Here's the drawing with two shaded views (mm, measured from the low corner). I have some questions. A direction names the side the tool comes from. Give positions to 0.01 mm unless a question says otherwise; leave off trailing zeros. Loops run counter-clockwise (first coordinate to the right, second up) from the corner with the lowest first, then second, coordinate; pieces in that order, holes last. Notation, with made-up numbers: (48, 26.25) - (64, 26.25) arc R14 cw to (64, 40.25) - close; hole circle Ø11 at (-28.75, 46). An arc over 180 degrees is marked (long way). Answer as a JSON object with one key per item and string values. Group by question number.
Item 1: Suppose I cut it at B-B on z = 21. Write out the boundary of the cut face in (x, y), and give its area (3 significant figures).
Item 2: Which directions (+Z, -Z, +X, -X, +Y, -Y) give clear straight access to the entire face, cutting with the end or side of a thin tool? Please do the marked faces 1, 2, 3, 4 and 5.
Item 3: Suppose I cut it at A-A on z = 7.5. Write out the boundary of the cut face in (x, y), and give its area (3 significant figures).
Item 4: Please list where these lines run through material, in increasing order: L1, parallel to Z at x = 22.5, y = 25; L2, parallel to X at y = 5, z = 81; L3, parallel to X at y = 10, z = 60.5.
Item 5: Will these pins go through, and if not, where does the flat tip stop? pin 1 (1 mm diameter, centred on x = 29.5, z = 21.5, fed in from +Y); pin 2 (10 mm diameter, centred on x = 19, z = 55.5, fed in from +Y); pin 3 (1 mm diameter, centred on x = 31, y = 37.5, fed in from -Z).
Item 6: Suppose I cut it at C-C on z = 68. Write out the boundary of the cut face in (x, y), and give its area (3 significant figures).
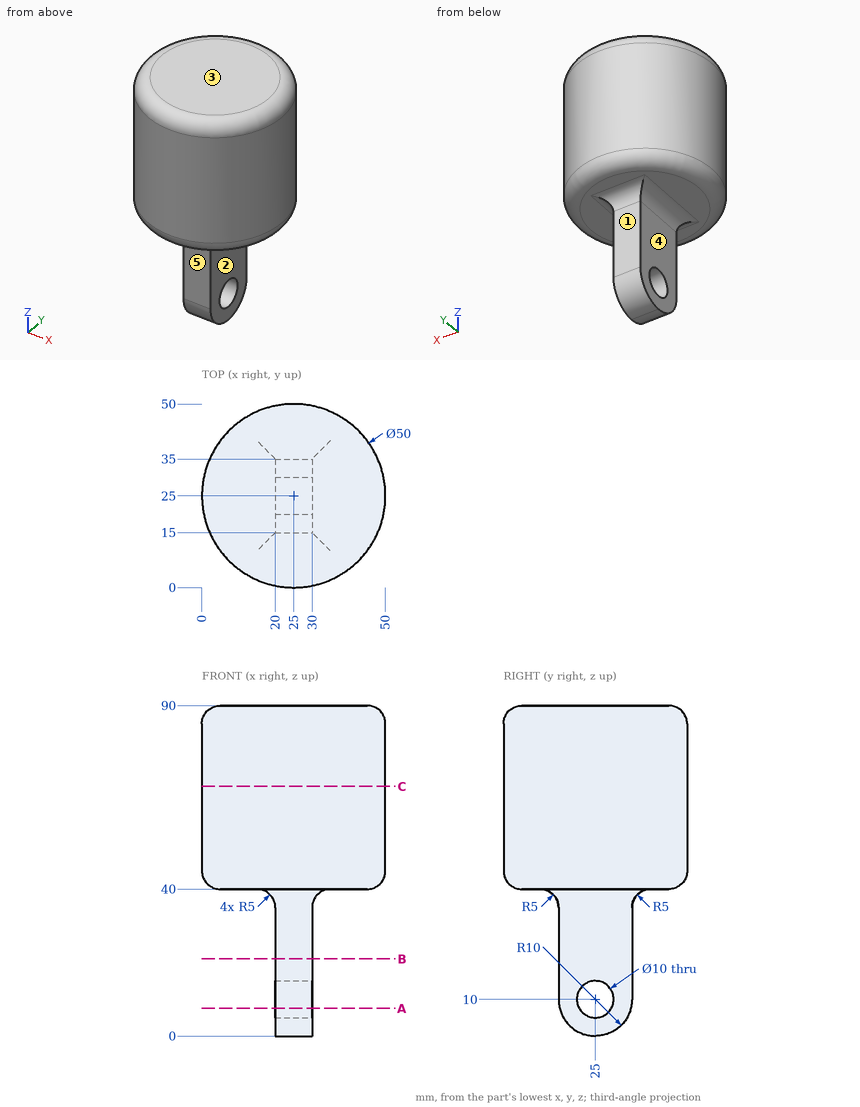
Worked out:
{
 "1": {"outline": "(20, 15) - (30, 15) - (30, 35) - (20, 35) - close", "area": "200 mm2"},
 "2": {"face 1": "-Z, +X, -X, +Y", "face 2": "-Z, +X, +Y, -Y", "face 3": "+Z, +X, -X, +Y, -Y", "face 4": "-Z, -X, +Y, -Y", "face 5": "-Z, +X, -X, -Y"},
 "3": {"outline": "(20, 15.32) - (30, 15.32) - (30, 20.67) - (20, 20.67) - close; (20, 29.33) - (30, 29.33) - (30, 34.68) - (20, 34.68) - close", "area": "107 mm2"},
 "4": {"L1": "z = 0 to 5, 15 to 90", "L2": "x = 10 to 40", "L3": "x = 5 to 45"},
 "5": {"pin 1": "stops at y = 35", "pin 2": "stops at y = 49.98", "pin 3": "stops at z = 39"},
 "6": {"outline": "circle Ø50 at (25, 25)", "area": "1,960 mm2"}
}
